```python
from build123d import *

# Parameters (mm, degrees)
BOSS_EXTRU_1_DEPTH      = 9
ESQUISSE2_W             = 19.623971562
ESQUISSE2_H             = 15.534154535
ESQUISSE2_R             = 3
ENL_V_MAT_EXTRU_1_DEPTH = 3
ENL_V_START             = -4
ESQUISSE3_W             = 11.267201257
ESQUISSE3_H             = 13.961169169
ESQUISSE3_R             = 3
ENL_V_MAT_EXTRU_2_DEPTH = 4
CHANFREIN1_SIZE         = 4
CHANFREIN1_SIZE_2       = 2.499477408


with BuildPart() as part:
    # Esquisse1 → Boss.-Extru.1 (new body)
    with BuildSketch(Plane.XY):
        Polygon((4.041451884, 0), (2.020725942, 3.5), (-2.020725942, 3.5), (-4.041451884, 0), (-2.020725942, -3.5), (2.020725942, -3.5), align=None)
    extrude(amount=BOSS_EXTRU_1_DEPTH)

    # Esquisse2 → Enlèv. mat.-Extru.1 (cut)
    with BuildSketch(Plane.XY.offset(9)):
        with Locations((0.327116653, -1.544441398)):
            Rectangle(ESQUISSE2_W, ESQUISSE2_H)
        Circle(ESQUISSE2_R, mode=Mode.SUBTRACT)
    extrude(amount=-ENL_V_MAT_EXTRU_1_DEPTH, mode=Mode.SUBTRACT)

    # Esquisse3 → Enlèv. mat.-Extru.2 (cut)
    with BuildSketch(Plane(origin=(0, 0, 0), x_dir=(-1, 0, 0), z_dir=(0, 0, -1)).offset(ENL_V_START)):
        with Locations((0.009770186, 0.039262349)):
            Rectangle(ESQUISSE3_W, ESQUISSE3_H)
        with Locations(Location((0, 0, 0), (0, 0, 180))):
            Circle(ESQUISSE3_R, mode=Mode.SUBTRACT)
    extrude(amount=ENL_V_MAT_EXTRU_2_DEPTH, mode=Mode.SUBTRACT)

    # Chanfrein1
    # the kernel refuses this chamfer: 4, 2.499477408 mm, written as the material it takes off along each edge
    with BuildSketch(Plane(origin=(0, 0, 0), x_dir=(1, 0, 0), z_dir=(0, 1, 0))) as chanfrein1_piece_1_section:
        Polygon((3, -CHANFREIN1_SIZE), (3 - CHANFREIN1_SIZE_2, 0), (3, 0), align=None)
    chanfrein1_piece_1 = revolve(axis=Axis((0, 0, 0), (0, 0, -1)), mode=Mode.PRIVATE)
    chanfrein1_piece_1 = split(chanfrein1_piece_1, bisect_by=Plane(origin=(-1.744026904, 0, 4), z_dir=(0, 0, -1)), keep=Keep.TOP, mode=Mode.PRIVATE)
    add(chanfrein1_piece_1, mode=Mode.SUBTRACT)

    # Esquisse4 → Enlèvement de matière-Révolution1 (revolve, cut)
    with BuildSketch(Plane(origin=(0, 0, 0), x_dir=(1, 0, 0), z_dir=(0, 1, 0))):
        Polygon((0, -9), (1, -9), (1, -6.108259821), (0.25, 0), (0, 0), align=None)
    revolve(axis=Axis((0, 0, 10.381605157), (0, 0, -1)), mode=Mode.SUBTRACT)


solid = part.part
```
Geometry: final body of the model. Coordinates: model frame, mm. A direction names the side the tool comes from. Coordinates: 2 decimals unless noted, no trailing zeros. Write each loop counter-clockwise with the first axis right and the second up, starting at its lowest first coordinate (ties: lowest second). Pieces come first, ordered by that corner, then holes. Notation, with made-up numbers: M 54.25,33.25 L 85.25,33.25 A26 ccw 85.25,69.25 Z; hole C 57,11.5 d3. An arc over 180 degrees is marked long. Answer as CSV lines item,"result". Start each with the question number.
Q1. Reachability of faces 5 (the flat face through (1, 3, 4)), 6 (the cylindrical face through (0, 1, 8)), 7 (the flat face through (0, 3.5, 5)) from +Z, -Z, +X, -X, +Y, -Y: full face, straight path, thin tool, end or side. Return the list, or none.
Q2. Line query: line 1 (Y direction, x = 0, z = 8); line 2 (Z direction, x = -0.25, y = 3.25); line 3 (X direction, y = 0, z = 1.5). Output: solid intervals per line, ascending. Write a range as from..to.
Q3. Cut plane D-D on z = 1.25. Return the cut outline in (x, y).
Q4. Mould query, pull axis X, two halves, no side actions, for faces 1 (the flat face through (-1, 3, 6)), 2 (the conical face through (-0.49, 0.38, 3.01)), 3 (the flat face through (3, -1.8, 5)), 4 (the flat face through (-3.045, -1.726, 4.986)). Classes: released by +X, released by -X, zero draft, split by the parting line, or undercut.
Q5. Cut plane B-B on z = 5.75. Return the cut outline in (x, y).
Q6. Pin query (flat end, axial travel): P1, Ø2, axis at y = 1, z = 2.5, coming from the +X side; P2, Ø3, axis at y = 2.5, z = 4, coming from the +X side. Return the tip coordinate at first contact, or that it passes through.
Q7. Cut plane A-A on x = 0. Return the cut outline in (y, z), then the cut area to 3 significant figures.
Q8. Cut plane C-C on z = 8.5. Return the cut outline in (x, y), then the cut area to 3 significant figures.
Findings below:
1,face 5,"-Z"
1,face 6,"+Z"
1,face 7,"+Z, -Z, +X, -X, +Y"
2,line 1,"y = -3..-1, 1..3"
2,line 2,"z = 4..6"
2,line 3,"x = -1.44..-0.43, 0.43..1.44"
3,outline,"C 0,0 d2.56; hole C 0,0 d0.81"
4,face 1,"zero draft"
4,face 2,"undercut"
4,face 3,"released by +X"
4,face 4,"released by -X"
5,outline,"M -4.04,0 L -2.02,-3.5 L 2.02,-3.5 L 4.04,0 L 2.02,3.5 L -2.02,3.5 Z; hole C 0,0 d1.91"
6,P1,"stops at x = 2.57"
6,P2,"stops at x = 3.46"
7,outline,"M -3.5,4 L -3,4 L -0.5,0 L -0.25,0 L -1,6.11 L -1,9 L -3,9 L -3,6 L -3.5,6 Z; M 0.25,0 L 0.5,0 L 3,4 L 3.5,4 L 3.5,6 L 3,6 L 3,9 L 1,9 L 1,6.11 Z"
7,area,"32.6 mm2"
8,outline,"C 0,0 d6; hole C 0,0 d2"
8,area,"25.1 mm2"
